Read the model definition and answer for the solid it produces. Units are mm, in the model's axes. Face numbers are marked on the shaded views. Give positions to 0.01 mm unless a question says otherwise; leave off trailing zeros. Order: outer loops, then holes, each group sorted by start corner. A loop starts at its lowest first (then second) coordinate and runs counter-clockwise, first axis right, second up. Notation, with made-up numbers: (-6, 83) - (21, 83) arc R32 cw to (21, 121) - close; hole circle Ø5 at (67.25, 84). An arc over 180 degrees is marked (long way). One line per item, written item: value. Start each with the question number.
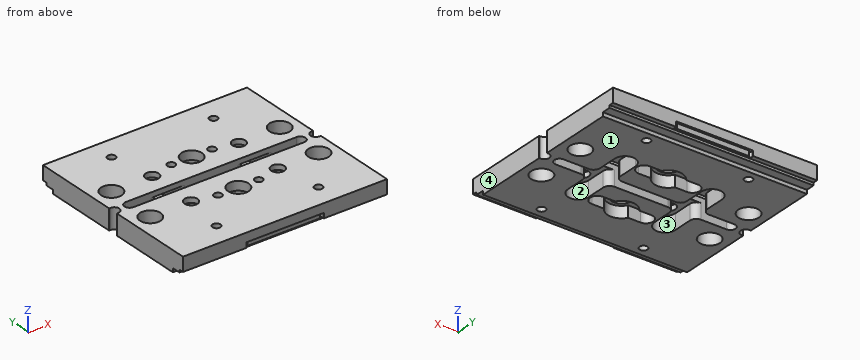
```python
from build123d import *

# Parameters (mm, degrees)
SKETCH_2_W           = 80
SKETCH_2_H           = 34
SKETCH_2_R           = 4.05
EXTRUDE_1_DEPTH      = 8
SKETCH_3_R           = 2.55
CUT_EXTRUDE_1_DEPTH  = 88.292611371
CUT_EXTRUDE_2_DEPTH  = 88.292611371
SKETCH_5_R           = 1.55
CUT_EXTRUDE_3_DEPTH  = 88.292611371
CUT_EXTRUDE_4_DEPTH  = 6
CUT_EXTRUDE_5_DEPTH  = 4.5
SKETCH_20_R          = 5.5
CUT_EXTRUDE_12_DEPTH = 4.5
SKETCH_25_R          = 1.55
CUT_EXTRUDE_13_DEPTH = 88.292611371
CUT_EXTRUDE_11_DEPTH = 2
EXTRUDE_2_DEPTH      = 8


with BuildPart() as part:
    # 草图2 → 凸台-拉伸1 (new body)
    with BuildSketch(Plane.XY):
        with Locations((40, 17)):
            Rectangle(SKETCH_2_W, SKETCH_2_H)
        with Locations((7, 8)):
            Circle(SKETCH_2_R, mode=Mode.SUBTRACT)
        with Locations((40, 10)):
            Circle(SKETCH_2_R, mode=Mode.SUBTRACT)
        with Locations((73, 8)):
            Circle(SKETCH_2_R, mode=Mode.SUBTRACT)
    extrude_1 = extrude(amount=EXTRUDE_1_DEPTH)

    # 草图3 → 切除-拉伸1 (cut, through all)
    with BuildSketch(Plane.XY.offset(8)):
        with Locations((23, 8)):
            Circle(SKETCH_3_R)
        with Locations((57, 8)):
            Circle(SKETCH_3_R)
    cut_extrude_1 = extrude(amount=-CUT_EXTRUDE_1_DEPTH, mode=Mode.SUBTRACT)

    # 草图4 → 切除-拉伸2 (cut, through all)
    with BuildSketch(Plane(origin=(80, 0, 0), x_dir=(0, 0, -1), z_dir=(1, 0, 0))):
        Polygon((-1.5, 32.2), (-2.5, 32.2), (-2.5, 34), (0, 34), (0, 28.8), (-1.5, 28.8), align=None)
    cut_extrude_2 = extrude(amount=-CUT_EXTRUDE_2_DEPTH, mode=Mode.SUBTRACT)

    # 草图5 → 切除-拉伸3 (cut, through all)
    with BuildSketch(Plane.XY.offset(8)):
        with Locations((48, 10)):
            Circle(SKETCH_5_R)
        with Locations((32, 10)):
            Circle(SKETCH_5_R)
    cut_extrude_3 = extrude(amount=-CUT_EXTRUDE_3_DEPTH, mode=Mode.SUBTRACT)

    # 草图7 → 切除-拉伸4 (cut)
    with BuildSketch(Plane(origin=(0, 0, 0), x_dir=(-1, 0, 0), z_dir=(0, 0, -1))):
        with BuildLine():
            Line((-27.05, 10), (-27.05, 2.5))
            ThreePointArc((-27.05, 2.5), (-27.782233047, 0.732233047), (-29.55, 0))
            Line((-29.55, 0), (-16.45, 0))
            ThreePointArc((-16.45, 0), (-18.217766953, 0.732233047), (-18.95, 2.5))
            Line((-18.95, 2.5), (-18.95, 10))
            ThreePointArc((-18.95, 10), (-23, 14.05), (-27.05, 10))
        make_face()
        with BuildLine():
            Line((-61.05, 2.5), (-61.05, 10))
            ThreePointArc((-61.05, 10), (-57, 14.05), (-52.95, 10))
            Line((-52.95, 10), (-52.95, 2.5))
            ThreePointArc((-52.95, 2.5), (-52.217766953, 0.732233047), (-50.45, 0))
            Line((-50.45, 0), (-63.55, 0))
            ThreePointArc((-63.55, 0), (-61.782233047, 0.732233047), (-61.05, 2.5))
        make_face()
    cut_extrude_4 = extrude(amount=-CUT_EXTRUDE_4_DEPTH, mode=Mode.SUBTRACT)

    # 草图8 → 切除-拉伸5 (cut)
    with BuildSketch(Plane(origin=(0, 0, 0), x_dir=(-1, 0, 0), z_dir=(0, 0, -1))):
        with BuildLine():
            Line((-30.5, 12.85), (-49.5, 12.85))
            ThreePointArc((-49.5, 12.85), (-52.35, 10), (-49.5, 7.15))
            Line((-49.5, 7.15), (-30.5, 7.15))
            ThreePointArc((-30.5, 7.15), (-27.65, 10), (-30.5, 12.85))
        make_face()
    cut_extrude_5 = extrude(amount=-CUT_EXTRUDE_5_DEPTH, mode=Mode.SUBTRACT)

    # 草图20 → 切除-拉伸12 (cut)
    with BuildSketch(Plane(origin=(0, 0, 0), x_dir=(-1, 0, 0), z_dir=(0, 0, -1))):
        with Locations((-40, 10)):
            Circle(SKETCH_20_R)
    cut_extrude_12 = extrude(amount=-CUT_EXTRUDE_12_DEPTH, mode=Mode.SUBTRACT)

    # 草图25 → 切除-拉伸13 (cut, through all)
    with BuildSketch(Plane(origin=(0, 0, 0), x_dir=(-1, 0, 0), z_dir=(0, 0, -1))):
        with Locations((-60, 25)):
            Circle(SKETCH_25_R)
        with Locations((-20, 25)):
            Circle(SKETCH_25_R)
    cut_extrude_13 = extrude(amount=-CUT_EXTRUDE_13_DEPTH, mode=Mode.SUBTRACT)

    # 草图19 → 切除-拉伸11 (cut)
    with BuildSketch(Plane(origin=(0, 0, 2.5), x_dir=(-1, 0, 0), z_dir=(0, 0, -1))):
        with BuildLine():
            Line((-25, 34), (-55.247938178, 34))
            Line((-55.247938178, 34), (-55.247938178, 33.2))
            ThreePointArc((-55.247938178, 33.2), (-54.747938178, 32.7), (-54.247938178, 33.2))
            Line((-54.247938178, 33.2), (-26, 33.2))
            ThreePointArc((-26, 33.2), (-25.5, 32.7), (-25, 33.2))
            Line((-25, 33.2), (-25, 34))
        make_face()
    cut_extrude_11 = extrude(amount=-CUT_EXTRUDE_11_DEPTH, mode=Mode.SUBTRACT)

    # 草图22 → 凸台-拉伸2 (add)
    with BuildSketch(Plane.XY.offset(8)):
        with BuildLine():
            Line((0.5, -4), (6.5, -4))
            ThreePointArc((6.5, -4), (4.5, -2), (6.5, 0))
            Line((6.5, 0), (0.5, 0))
            ThreePointArc((0.5, 0), (2.5, -2), (0.5, -4))
        make_face()
        with BuildLine():
            Line((79.5, 0), (73.5, 0))
            ThreePointArc((73.5, 0), (75.5, -2), (73.5, -4))
            Line((73.5, -4), (79.5, -4))
            ThreePointArc((79.5, -4), (77.5, -2), (79.5, 0))
        make_face()
    extrude(amount=-EXTRUDE_2_DEPTH)

    # 镜向2: 凸台-拉伸1, 切除-拉伸1, 切除-拉伸2, 切除-拉伸3, 切除-拉伸4, 切除-拉伸5, 切除-拉伸12, 切除-拉伸13, 切除-拉伸11 across plane
    add(extrude_1.mirror(Plane(origin=(0, -2, 0), x_dir=(0, 0, 1), z_dir=(0, -1, 0))))
    add(cut_extrude_1.mirror(Plane(origin=(0, -2, 0), x_dir=(0, 0, 1), z_dir=(0, -1, 0))), mode=Mode.SUBTRACT)
    add(cut_extrude_2.mirror(Plane(origin=(0, -2, 0), x_dir=(0, 0, 1), z_dir=(0, -1, 0))), mode=Mode.SUBTRACT)
    add(cut_extrude_3.mirror(Plane(origin=(0, -2, 0), x_dir=(0, 0, 1), z_dir=(0, -1, 0))), mode=Mode.SUBTRACT)
    add(cut_extrude_4.mirror(Plane(origin=(0, -2, 0), x_dir=(0, 0, 1), z_dir=(0, -1, 0))), mode=Mode.SUBTRACT)
    add(cut_extrude_5.mirror(Plane(origin=(0, -2, 0), x_dir=(0, 0, 1), z_dir=(0, -1, 0))), mode=Mode.SUBTRACT)
    add(cut_extrude_12.mirror(Plane(origin=(0, -2, 0), x_dir=(0, 0, 1), z_dir=(0, -1, 0))), mode=Mode.SUBTRACT)
    add(cut_extrude_13.mirror(Plane(origin=(0, -2, 0), x_dir=(0, 0, 1), z_dir=(0, -1, 0))), mode=Mode.SUBTRACT)
    add(cut_extrude_11.mirror(Plane(origin=(0, -2, 0), x_dir=(0, 0, 1), z_dir=(0, -1, 0))), mode=Mode.SUBTRACT)


solid = part.part
```
1) Section A-A on x = 12.5 is taken. Write down the section's boundary in (y, z), plus the area to 3 significant figures.
2) Each of these flat-tipped pins is pushed along its axis until it touches: pin 1 (1.3 mm diameter, centred on x = 32.5, z = 3, fed in from +Y); pin 2 (2 mm diameter, centred on x = 23, y = -37, fed in from -Z); pin 3 (0.5 mm diameter, centred on x = 57, z = 2, fed in from -Y). Where does it stop, or does it pass through?
3) The mould has two halves that part along X. Classify the marked faces 1, 2, 3 and 4: +X half, -X half, draft (parallel to the pull), parting line (faces both ways), or undercut.
4) Section B-B on x = 40 is taken. Give the number of separate pieces and of enclosed holes in the cut face, plus the area to 3 significant figures.
5) Find the intervals of material crossed by probe 1 along Y at (x, z) = (57, 7.1); probe 2 along Y at (x, z) = (40, 4); probe 3 along X at (y, z) = (1, 1.5), in increasing order. Write a range as from..to.
Solved:
1. outline: (-38, 2.5) - (-36.2, 2.5) - (-36.2, 1.5) - (-32.8, 1.5) - (-32.8, 0) - (-4, 0) - (-4, 8) - (-38, 8) - close; (0, 0) - (28.8, 0) - (28.8, 1.5) - (32.2, 1.5) - (32.2, 2.5) - (34, 2.5) - (34, 8) - (0, 8) - close
1. area: 525 mm2
2. pin 1: stops at y = 33.2
2. pin 2: stops at z = 1.5
2. pin 3: stops at y = -36.2
3. face 1: draft
3. face 2: undercut
3. face 3: undercut
3. face 4: +X half
4. separate pieces: 4
4. enclosed holes: 0
4. area: 366 mm2
5. probe 1: y = -38..-14.55, -9.45..-4, 0..5.45, 10.55..34
5. probe 2: y = -37.2..-19.5, -8.5..-4, 0..4.5, 15.5..33.2
5. probe 3: x = 0..18.45, 27.55..52.45, 61.55..80
